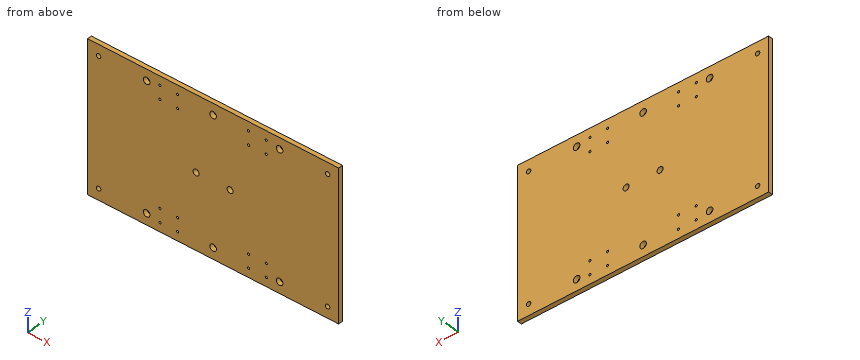
from build123d import *

# Parameters (mm, degrees)
SKETCH1_W           = 340
SKETCH1_H           = 200
SKETCH1_R           = 4.1
SKETCH1_R_2         = 1.5
SKETCH1_R_3         = 3
SKETCH1_R_4         = 4.5
BOSS_EXTRUDE1_DEPTH = 6


with BuildPart() as part:
    # Sketch1 → Boss-Extrude1 (new body)
    with BuildSketch(Plane(origin=(0, 0, 0), x_dir=(1, 0, 0), z_dir=(0, 1, 0))):
        Rectangle(SKETCH1_W, SKETCH1_H)
        with Locations((-23, 0)):
            Circle(SKETCH1_R, mode=Mode.SUBTRACT)
        with Locations((23, 0)):
            Circle(SKETCH1_R, mode=Mode.SUBTRACT)
        with Locations((72, 88)):
            Circle(SKETCH1_R_2, mode=Mode.SUBTRACT)
        with Locations((48, 88)):
            Circle(SKETCH1_R_2, mode=Mode.SUBTRACT)
        with Locations((72, 70)):
            Circle(SKETCH1_R_2, mode=Mode.SUBTRACT)
        with Locations((48, 70)):
            Circle(SKETCH1_R_2, mode=Mode.SUBTRACT)
        with Locations((-48, 70)):
            Circle(SKETCH1_R_2, mode=Mode.SUBTRACT)
        with Locations((-72, 70)):
            Circle(SKETCH1_R_2, mode=Mode.SUBTRACT)
        with Locations((-48, 88)):
            Circle(SKETCH1_R_2, mode=Mode.SUBTRACT)
        with Locations((-72, 88)):
            Circle(SKETCH1_R_2, mode=Mode.SUBTRACT)
        with Locations((-72, -88)):
            Circle(SKETCH1_R_2, mode=Mode.SUBTRACT)
        with Locations((-48, -88)):
            Circle(SKETCH1_R_2, mode=Mode.SUBTRACT)
        with Locations((-72, -70)):
            Circle(SKETCH1_R_2, mode=Mode.SUBTRACT)
        with Locations((-48, -70)):
            Circle(SKETCH1_R_2, mode=Mode.SUBTRACT)
        with Locations((48, -70)):
            Circle(SKETCH1_R_2, mode=Mode.SUBTRACT)
        with Locations((72, -70)):
            Circle(SKETCH1_R_2, mode=Mode.SUBTRACT)
        with Locations((48, -88)):
            Circle(SKETCH1_R_2, mode=Mode.SUBTRACT)
        with Locations((72, -88)):
            Circle(SKETCH1_R_2, mode=Mode.SUBTRACT)
        with Locations((155, 85)):
            Circle(SKETCH1_R_3, mode=Mode.SUBTRACT)
        with Locations((-155, 85)):
            Circle(SKETCH1_R_3, mode=Mode.SUBTRACT)
        with Locations((155, -85)):
            Circle(SKETCH1_R_3, mode=Mode.SUBTRACT)
        with Locations((-155, -85)):
            Circle(SKETCH1_R_3, mode=Mode.SUBTRACT)
        with Locations((0, 85)):
            Circle(SKETCH1_R_4, mode=Mode.SUBTRACT)
        with Locations((0, -85)):
            Circle(SKETCH1_R_4, mode=Mode.SUBTRACT)
        with Locations((90, 85)):
            Circle(SKETCH1_R_4, mode=Mode.SUBTRACT)
        with Locations((90, -85)):
            Circle(SKETCH1_R_4, mode=Mode.SUBTRACT)
        with Locations((-90, -85)):
            Circle(SKETCH1_R_4, mode=Mode.SUBTRACT)
        with Locations((-90, 85)):
            Circle(SKETCH1_R_4, mode=Mode.SUBTRACT)
    extrude(amount=BOSS_EXTRUDE1_DEPTH)


solid = part.part
Geometry: final body of the model. Coordinates: model frame, mm. Give positions to 0.01 mm unless a question says otherwise; leave off trailing zeros. Write each loop counter-clockwise with the first axis right and the second up, starting at its lowest first coordinate (ties: lowest second). Pieces come first, ordered by that corner, then holes. Notation, with made-up numbers: M 67.25,81.25 L 80.25,81.25 A16 ccw 80.25,109.25 Z; hole C 20.5,1 d11. An arc over 180 degrees is marked long. Answer in a Markdown table with one row per item. Add a question column.
(1) Ray query, line 1 (X direction, y = 2, z = -85); line 2 (X direction, y = 3.05, z = -70); line 3 (Z direction, x = -48, y = 2.55). Return the intervals inside material, ascending.
(2) First-contact query: pin 1 (5 mm diameter, centred on x = 72, z = -88, fed in from -Y). Flat tip, straight axial feed; report the tip coordinate or a pass-through.
(3) Section A-A on x = 23. Return loops of the section in (y, z).
(4) Section B-B on z = 0. Return loops of the section in (x, y).
Result set:
| question | item | result |
|---|---|---|
| 1 | line 1 | x = -170 to -158, -152 to -94.5, -85.5 to -4.5, 4.5 to 85.5, 94.5 to 152, 158 to 170 |
| 1 | line 2 | x = -170 to -73.5, -70.5 to -49.5, -46.5 to 46.5, 49.5 to 70.5, 73.5 to 170 |
| 1 | line 3 | z = -100 to -89.5, -86.5 to -71.5, -68.5 to 68.5, 71.5 to 86.5, 89.5 to 100 |
| 2 | pin 1 | stops at y = 0 |
| 3 | outline | M 0,-100 L 6,-100 L 6,-4.1 L 0,-4.1 Z; M 0,4.1 L 6,4.1 L 6,100 L 0,100 Z |
| 4 | outline | M -170,0 L -27.1,0 L -27.1,6 L -170,6 Z; M -18.9,0 L 18.9,0 L 18.9,6 L -18.9,6 Z; M 27.1,0 L 170,0 L 170,6 L 27.1,6 Z |
